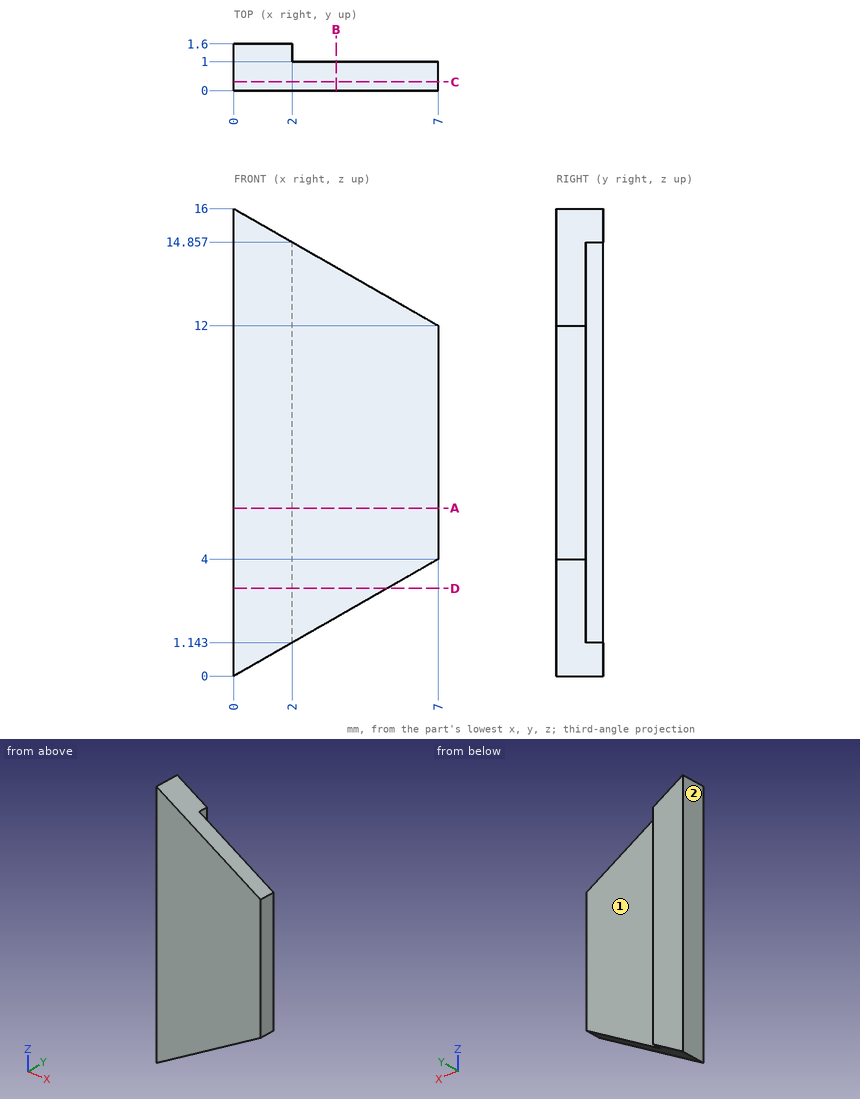
Job drawing, mm, ordinate dimensions from the low corner. One solid piece. A direction names the side the tool comes from. Coordinates: 2 decimals unless noted, no trailing zeros. Loops run counter-clockwise (first coordinate to the right, second up) from the corner with the lowest first, then second, coordinate; pieces in that order, holes last. Notation, with made-up numbers: (8, 4.5) -> (39, 4.5) arc R30 cw to (39, 27.5) -> close; hole circle Ø7 at (42, 43.5). An arc over 180 degrees is marked (long way). One line per item, written item: value.
1. Flat gauge pins, fed straight in: P1, Ø0.5, axis at y = 1.5, z = 5, coming from the +X side; P2, Ø4, axis at x = 6, z = 10.5, coming from the +Y side. Where does each tip first touch, or does it go through?
Answers:
P1: stops at x = 2
P2: stops at y = 1
2. Slice it at A-A on z = 5.75. Write the cut outline in (x, y), and give its area (3 significant figures).
Answers:
outline: (0, 0) -> (7, 0) -> (7, 1) -> (2, 1) -> (2, 1.6) -> (0, 1.6) -> close
area: 8.20 mm^2
3. Slice it at C-C on y = 0.3. Write the cut outline in (x, z), and give its area (3 significant figures).
Answers:
outline: (0, 0) -> (7, 4) -> (7, 12) -> (0, 16) -> close
area: 84.0 mm^2
4. Slice it at B-B on x = 3.5. Write the cut outline in (y, z), and give its area (3 significant figures).
Answers:
outline: (0, 2) -> (1, 2) -> (1, 14) -> (0, 14) -> close
area: 12.0 mm^2
5. Drill centre lines: line 1 (Y direction, x = 2.75, z = 5.5); line 2 (X direction, y = 1.25, z = 8); line 3 (X direction, y = 0.15, z = 3.25). Where is each one in solid material? Low to high. Write a range as [from, to].
Answers:
line 1: y = [0, 1]
line 2: x = [0, 2]
line 3: x = [0, 5.69]
6. Slice it at D-D on z = 3. Write the cut outline in (x, y), and give its area (3 significant figures).
Answers:
outline: (0, 0) -> (5.25, 0) -> (5.25, 1) -> (2, 1) -> (2, 1.6) -> (0, 1.6) -> close
area: 6.45 mm^2
7. Which spindle directions (+Z, -Z, +X, -X, +Y, -Y) get a long thin tool onto all of the face, cutting with end or side? Do the marked faces 1 and 2. Say none if no direction does.
Answers:
face 1: +Z, -Z, +X, +Y
face 2: +Z, -Z, -X, +Y, -Y
